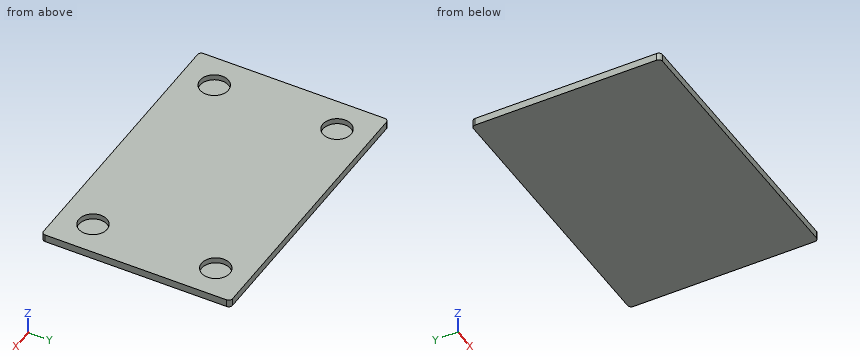
from build123d import *

# Parameters (mm, degrees)
F0_W     = 150
F0_H     = 100
F1_DEPTH = 4
F2_R     = 7.5
F3_DEPTH = 3
F4_R     = 2


with BuildPart() as f1:
    # F0 (on Top) → F1 (new body)
    with BuildSketch(Plane.XY):
        with Locations((75, 50)):
            Rectangle(F0_W, F0_H)
    extrude(amount=F1_DEPTH)

    # F2 (on face) → F3 (cut)
    with BuildSketch(Plane.XY.offset(4)):
        with Locations((17.5, 82.5)):
            Circle(F2_R)
        with Locations((132.5, 82.5)):
            Circle(F2_R)
        with Locations((132.5, 17.5)):
            Circle(F2_R)
        with Locations((17.5, 17.5)):
            Circle(F2_R)
    extrude(amount=-F3_DEPTH, mode=Mode.SUBTRACT)

    # F4
    f4_edges = [f1.edges().sort_by_distance(p)[0] for p in [
        (0, 0, 2),
        (0, 100, 2),
        (150, 100, 2),
        (150, 0, 2),
    ]]
    fillet(f4_edges, radius=F4_R)


solid = f1.part
Read the model definition and answer for the solid it produces. Units are mm, in the model's axes. Round coordinates to 2 decimals unless told otherwise and drop trailing zeros. Write each loop counter-clockwise with the first axis right and the second up, starting at its lowest first coordinate (ties: lowest second). Pieces come first, ordered by that corner, then holes. Notation, with made-up numbers: (24.5, 83) - (37.5, 83) arc R32 cw to (37.5, 120) - close; hole circle Ø9 at (8, 71). An arc over 180 degrees is marked (long way). Use a Markdown table: item, result.
(1) The part is cut by section A-A (x = 132.5). Write down the section's boundary in (y, z), then the cut area to 3 significant figures.
Reported:
| item | result |
|---|---|
| outline | (0, 0) - (100, 0) - (100, 4) - (90, 4) - (90, 1) - (75, 1) - (75, 4) - (25, 4) - (25, 1) - (10, 1) - (10, 4) - (0, 4) - close |
| area | 310 mm2 |
(2) The part is cut by section B-B (y = 17.5). Write down the section's boundary in (x, z), then the cut area to 3 significant figures.
Reported:
| item | result |
|---|---|
| outline | (0, 0) - (150, 0) - (150, 4) - (140, 4) - (140, 1) - (125, 1) - (125, 4) - (25, 4) - (25, 1) - (10, 1) - (10, 4) - (0, 4) - close |
| area | 510 mm2 |
(3) Straight lines are drawn through the part: line 1 along Y through (x, z) = (132.5, 2); line 2 along Y through (x, z) = (129, 3.85); line 3 along Z through (x, y) = (11, 79.5). For each, find the intervals that lie inside material, in ascending order. Write a range as [from, to].
Reported:
| item | result |
|---|---|
| line 1 | [0, 10], [25, 75], [90, 100] |
| line 2 | [0, 10.87], [24.13, 75.87], [89.13, 100] |
| line 3 | [0, 1] |
(4) This flat-tipped pin is pushed along its axis until it touches: pin 1 Ø9 at (x, y) = (132.5, 17.5) entering from +Z. Where does it stop, or does it pass through?
Reported:
| item | result |
|---|---|
| pin 1 | z = 1 |
